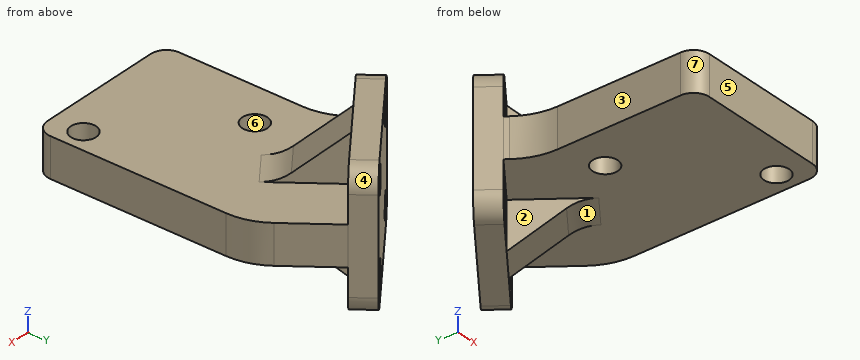
from build123d import *

# Parameters (mm, degrees)
SKETCH_1_R      = 1.6
EXTRUDE_1_DEPTH = 5
SKETCH_2_R      = 1.6
EXTRUDE_2_DEPTH = 3
EXTRUDE_START   = -7.5
EXTRUDE_4_DEPTH = 5
FILLET_1_R      = 5


with BuildPart() as part:
    # 草图1 → 凸台-拉伸1 (new body)
    with BuildSketch(Plane.XY):
        with BuildLine():
            Line((0, 2), (0, 17.705362587))
            ThreePointArc((0, 17.705362587), (-0.413410758, 20.243799839), (-1.61091592, 22.519882772))
            Line((-1.61091592, 22.519882772), (-1.972710201, 23))
            Line((-1.972710201, 23), (14, 35.036300463))
            Line((14, 35.036300463), (18.38908408, 29.211789163))
            ThreePointArc((18.38908408, 29.211789163), (19.586589242, 26.935706229), (20, 24.397268977))
            Line((20, 24.397268977), (20, 2))
            ThreePointArc((20, 2), (19.414213562, 0.585786438), (18, 0))
            Line((18, 0), (2, 0))
            ThreePointArc((2, 0), (0.585786438, 0.585786438), (0, 2))
        make_face()
        with Locations((5.3, 16)):
            Circle(SKETCH_1_R, mode=Mode.SUBTRACT)
        with Locations((17.3, 4)):
            Circle(SKETCH_1_R, mode=Mode.SUBTRACT)
    extrude(amount=EXTRUDE_1_DEPTH)

    # 草图2 → 凸台-拉伸2 (add)
    with BuildSketch(Plane(origin=(-11.768988292, 15.617974969, 0), x_dir=(0.79863551, 0.601815023, 0), z_dir=(-0.601815023, 0.79863551, 0))):
        with BuildLine():
            Line((29.766269115, -11), (14.766269115, -11))
            ThreePointArc((14.766269115, -11), (12.998502162, -10.267766953), (12.266269115, -8.5))
            Line((12.266269115, -8.5), (12.266269115, 3.5))
            ThreePointArc((12.266269115, 3.5), (12.998502162, 5.267766953), (14.766269115, 6))
            Line((14.766269115, 6), (29.766269115, 6))
            ThreePointArc((29.766269115, 6), (31.534036068, 5.267766953), (32.266269115, 3.5))
            Line((32.266269115, 3.5), (32.266269115, -8.5))
            ThreePointArc((32.266269115, -8.5), (31.534036068, -10.267766953), (29.766269115, -11))
        make_face()
        with Locations((16.016269115, 3)):
            Circle(SKETCH_2_R, mode=Mode.SUBTRACT)
        with Locations((28.516269115, 3)):
            Circle(SKETCH_2_R, mode=Mode.SUBTRACT)
        with Locations((28.516269115, -8)):
            Circle(SKETCH_2_R, mode=Mode.SUBTRACT)
        with Locations((16.016269115, -8)):
            Circle(SKETCH_2_R, mode=Mode.SUBTRACT)
    extrude(amount=EXTRUDE_2_DEPTH)

    # 草图6 → 凸台-拉伸4 (add)
    with BuildSketch(Plane(origin=(25.768988292, 19.418325494, 0), x_dir=(0, 0, -1), z_dir=(0.79863551, 0.601815023, 0)).offset(EXTRUDE_START)):
        Polygon((-11, 19.555823366), (-5, 12.262745076), (-5, 19.555823366), align=None)
        Polygon((0, 12.262745076), (6, 19.555823366), (0, 19.555823366), align=None)
    extrude(amount=-EXTRUDE_4_DEPTH)

    # 圆角1
    fillet_1_edges = [part.edges().sort_by_distance(p)[0] for p in [
        (10.40272898, 23.193638931, 5),
        (10.40272898, 23.193638931, 0),
    ]]
    fillet(fillet_1_edges, radius=FILLET_1_R)


solid = part.part
The listing builds one solid part. Answer for the finished solid, in the listing's coordinates (mm). Face numbers are marked on the shaded views. A direction names the side the tool comes from. Give positions to 0.01 mm unless a question says otherwise; leave off trailing zeros. Loops run counter-clockwise (first coordinate to the right, second up) from the corner with the lowest first, then second, coordinate; pieces in that order, holes last. Notation, with made-up numbers: (-29.5, 39) - (22.5, 39) arc R14 cw to (22.5, 58) - close; hole circle Ø2 at (-23, 19.25). An arc over 180 degrees is marked (long way). Use one line per item in the form item = value.
1. Section A-A on z = 0.75 is taken. Give the vertices of the cut face in (x, y).
Calculated:
outline = (-3.78, 25.4) - (-1.61, 22.52) arc R8 cw to (0, 17.71) - (0, 2) arc R2 ccw to (2, 0) - (18, 0) arc R2 ccw to (20, 2) - (20, 24.4) arc R8 ccw to (18.39, 29.21) - (12.19, 37.43) - close; hole circle Ø3.2 at (5.3, 16); hole circle Ø3.2 at (17.3, 4)
2. Given pin 1 Ø4 at (y, z) = (11, 1.5) entering from -X; pin 2 Ø4 at (x, y) = (6.5, 23) entering from -Z; pin 3 Ø6 at (x, z) = (14, 8.5) entering from -Y, each flat-ended and moving along its own axis, determine where each tip first touches the part or whether it passes through.
Calculated:
pin_1 = 0
pin_2 = -3.34
pin_3 = 32.93
3. Find the intervals of material crossed by line 1 along Z through (x, y) = (13.25, 18); line 2 along X through (y, z) = (6, 1.25); line 3 along Y through (x, z) = (5.3, 3.8), in increasing order. Write a range as [from, to].
Calculated:
line_1 = [0, 5]
line_2 = [0, 20]
line_3 = [0, 14.4], [17.6, 32.24]
4. Section B-B on y = 16 is taken. Give the vertices of the cut face in (x, z).
Calculated:
outline = (0, 0) - (3.7, 0) - (3.7, 5) - (0, 5) - close; (6.9, 0) - (20, 0) - (20, 5) - (6.9, 5) - close
5. Section C-C on x = 17.3 is taken. Give the vertices of the cut face in (y, z).
Calculated:
outline = (0, 0) - (2.4, 0) - (2.4, 5) - (0, 5) - close; (5.6, 0) - (30.66, 0) - (30.66, 5) - (5.6, 5) - close
6. Section D-D on z = 9 is taken. Give the vertices of the cut face in (x, y), then the cut area to 3 significant figures.
Calculated:
outline = (-3.74, 25.43) - (-1.93, 23.03) - (0.02, 24.51) - (-1.78, 26.9) - close; (0.21, 28.4) - (2.02, 26.01) - (4.02, 27.51) - (5.48, 25.57) - (9.47, 28.58) - (8.01, 30.52) - (10.01, 32.03) - (8.2, 34.42) - close; (10.2, 35.93) - (12, 33.53) - (13.96, 35.01) - (12.15, 37.4) - close
area = 56.9 mm^2
7. Which of the six approach directions +Z, -Z, +X, -X, +Y, -Y give full straight-line access (tool end or side, diameter ignored) to the marked faces 1, 2 and 3?
Calculated:
face_1 = -Z, +X, -Y
face_2 = -Z, -Y
face_3 = +Z, -Z, -X, -Y
8. The mould has two halves that part along X. Classify the marked faces 4, 5, 6 and 7: pulls with the +X half, pulls with the -X half, needs draft (parallel to the pull), parting line crosses it, or undercut.
Calculated:
face_4 = pulls with the +X half
face_5 = needs draft
face_6 = undercut
face_7 = pulls with the -X half
